Study the drawing (mm; zero at the part's minimum x, y, z) and answer. Round coordinates to 2 decimals unless told otherwise and drop trailing zeros. Write each loop counter-clockwise with the first axis right and the second up, starting at its lowest first coordinate (ties: lowest second). Pieces come first, ordered by that corner, then holes.
(1) A cutting plane is placed at A-A, the plane z = 23.5. Give the vertices of the cut face in (x, y).
(2) A cutting plane is placed at B-B, the plane x = 1.75. Give the vertices of the cut face in (y, z).
(3) This flat-tipped pin is pushed along its axis until it touches: pin 1 Ø2 at (y, z) = (1, 29.5) entering from +X. Where does it stop, or does it pass through?
(4) Find the intervals of material crossed by probe 1 along X at (y, z) = (4.25, 32); probe 2 along Y at (x, z) = (1.5, 65.5), in increasing order.
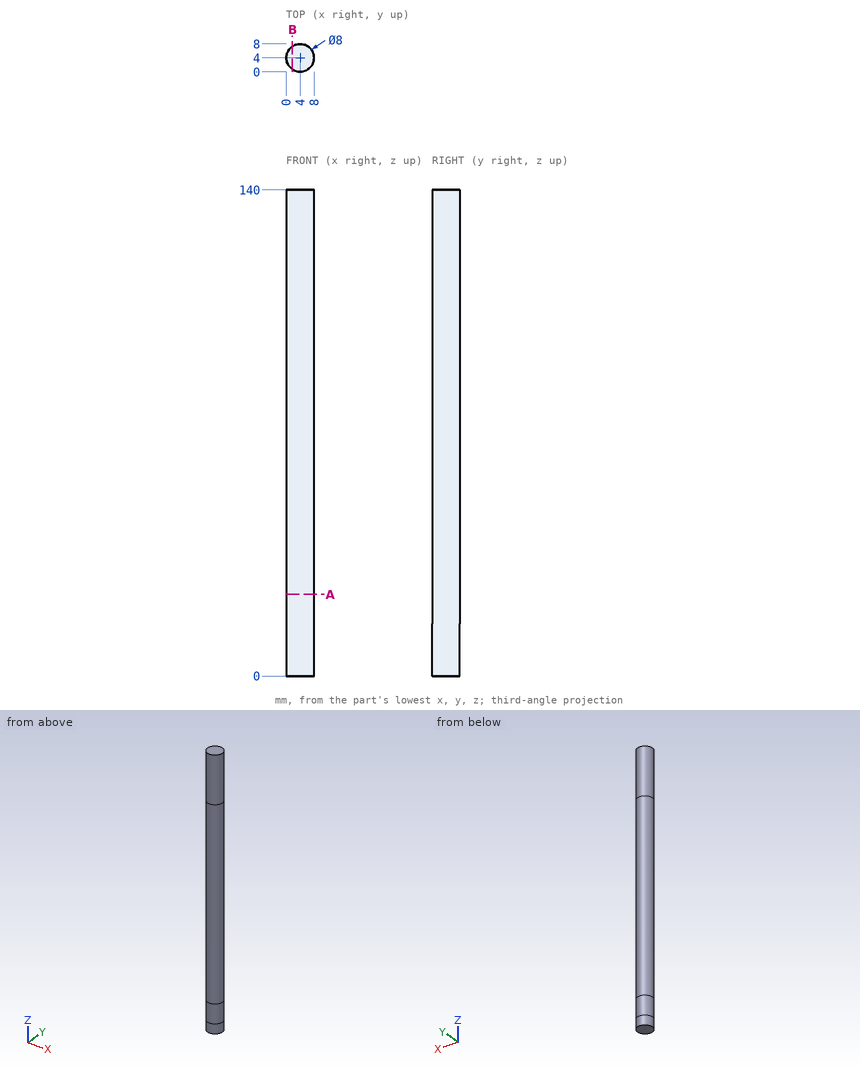
Solutions:
1. outline: circle Ø8 at (4, 4)
2. outline: (0.69, 0) - (7.31, 0) - (7.31, 140) - (0.69, 140) - close
3. pin 1: stops at x = 7.46
4. probe 1: x = 0.01 to 7.99
4. probe 2: y = 0.88 to 7.12
